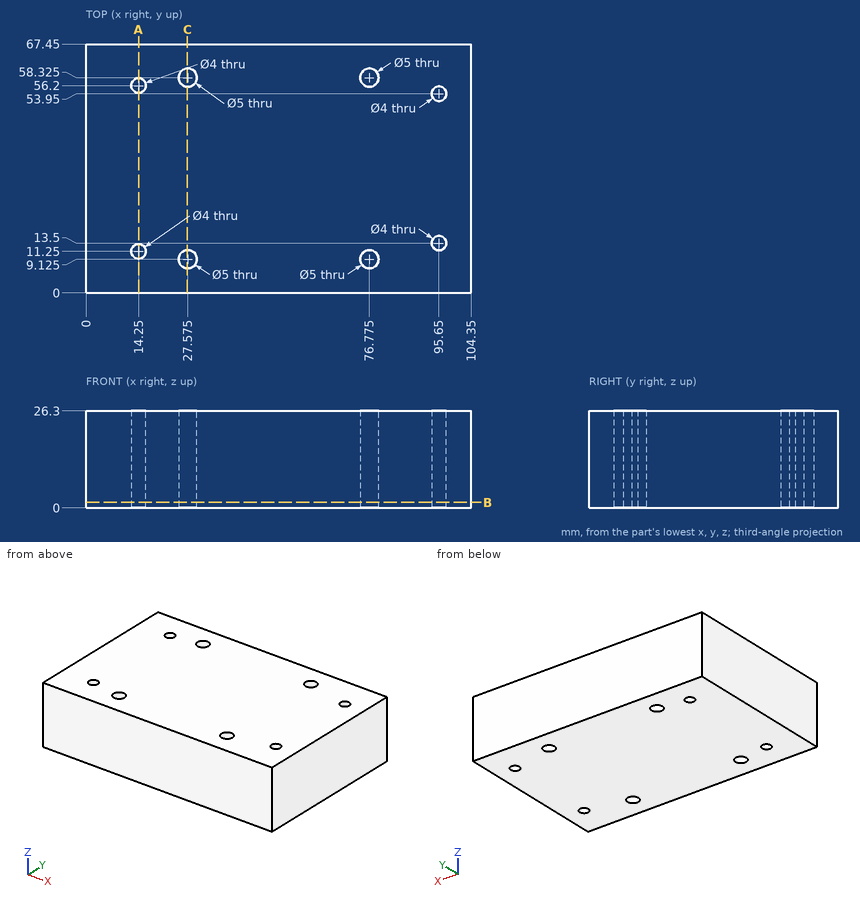
Could you check a few things on this drawing? It's one solid part, dimensions in mm from its lowest x, y, z. Coordinates: 2 decimals unless noted, no trailing zeros. Order: outer loops, then holes, each group sorted by start corner. A loop starts at its lowest first (then second) coordinate and runs counter-clockwise, first axis right, second up. Notation, with made-up numbers: (81.25, 85.5) -> (96.25, 85.5) arc R29 cw to (96.25, 116.5) -> close; hole circle Ø2 at (27, 18). An arc over 180 degrees is marked (long way). Answer in a Markdown table with one row per item.
(1) Please list where these lines run through material, in increasing order: probe 1 along Y at (x, z) = (95.65, 6); probe 2 along Y at (x, z) = (14.25, 19.5); probe 3 along X at (y, z) = (13.5, 6).
Answer key:
| item | result |
|---|---|
| probe 1 | 0 to 11.5, 15.5 to 51.95, 55.95 to 67.45 |
| probe 2 | 0 to 9.25, 13.25 to 54.2, 58.2 to 67.45 |
| probe 3 | 0 to 93.65, 97.65 to 104.35 |
(2) I want a section at B-B on z = 1.5. Count the separate pieces of the cut face and the enclosed holes in it, then the cut area to 3 significant figures.
Answer key:
| item | result |
|---|---|
| separate pieces | 1 |
| enclosed holes | 8 |
| area | 6,910 mm^2 |
(3) Will this pin go through, and if not, where does the flat tip stop? pin 1 Ø10 at (x, y) = (37.5, 31.5) entering from -Z.
Answer key:
| item | result |
|---|---|
| pin 1 | z = 0 |
(4) I want a section at C-C on x = 27.5. List the corners of the cut face in (y, z) for me.
Answer key:
| item | result |
|---|---|
| outline | (0, 0) -> (6.63, 0) -> (6.63, 26.3) -> (0, 26.3) -> close; (11.62, 0) -> (55.83, 0) -> (55.83, 26.3) -> (11.62, 26.3) -> close; (60.82, 0) -> (67.45, 0) -> (67.45, 26.3) -> (60.82, 26.3) -> close |
(5) I want a section at A-A on x = 14.25. List the corners of the cut face in (y, z) for me, then the cut area to 3 significant figures.
Answer key:
| item | result |
|---|---|
| outline | (0, 0) -> (9.25, 0) -> (9.25, 26.3) -> (0, 26.3) -> close; (13.25, 0) -> (54.2, 0) -> (54.2, 26.3) -> (13.25, 26.3) -> close; (58.2, 0) -> (67.45, 0) -> (67.45, 26.3) -> (58.2, 26.3) -> close |
| area | 1,560 mm^2 |
